```python
from build123d import *

# Parameters (mm, degrees)
SKETCH_2_W          = 75
SKETCH_2_H          = 40
EXTRUDE_1_DEPTH     = 2
SKETCH_3_R          = 5.05
SKETCH_3_R_2        = 1.25
CUT_EXTRUDE_1_DEPTH = 86.023526156
FILLET_1_R          = 20
SKETCH_7_W          = 2
SKETCH_7_H          = 40
EXTRUDE_3_DEPTH     = 10
SKETCH_10_R         = 1.5
CUT_EXTRUDE_4_DEPTH = 84.839131675


with BuildPart() as part:
    # 草图2 → 凸台-拉伸1 (new body)
    with BuildSketch(Plane.XY):
        with Locations((37.5, 20)):
            Rectangle(SKETCH_2_W, SKETCH_2_H)
    extrude(amount=EXTRUDE_1_DEPTH)

    # 草图3 → 切除-拉伸1 (cut, through all)
    with BuildSketch(Plane(origin=(0, 0, 0), x_dir=(-1, 0, 0), z_dir=(0, 0, -1))):
        with Locations((-26, 20)):
            Circle(SKETCH_3_R)
        with Locations((-16, 10.202041029)):
            Circle(SKETCH_3_R_2)
        with BuildLine():
            ThreePointArc((-36.446428571, 32.447274003), (-39.704318392, 11.267637352), (-19.131116422, 5.273121906))
            ThreePointArc((-19.131116422, 5.273121906), (-18.043086412, 8.263304292), (-21.033268797, 9.351334301))
            ThreePointArc((-21.033268797, 9.351334301), (-35.909276376, 13.685830085), (-33.553571429, 29.000336587))
            ThreePointArc((-33.553571429, 29.000336587), (-33.276531292, 32.170233866), (-36.446428571, 32.447274003))
        make_face()
    extrude(amount=-CUT_EXTRUDE_1_DEPTH, mode=Mode.SUBTRACT)

    # 圆角1
    fillet_1_edges = [part.edges().sort_by_distance(p)[0] for p in [
        (0, 40, 1),
        (0, 0, 1),
    ]]
    fillet(fillet_1_edges, radius=FILLET_1_R - 0.0001)  # a hair under: the kernel refuses the full size

    # 草图7 → 凸台-拉伸3 (add)
    with BuildSketch(Plane(origin=(0, 0, 0), x_dir=(-1, 0, 0), z_dir=(0, 0, -1))):
        with Locations((-74, 20)):
            Rectangle(SKETCH_7_W, SKETCH_7_H)
    extrude(amount=EXTRUDE_3_DEPTH)

    # 草图10 → 切除-拉伸4 (cut, through all)
    with BuildSketch(Plane.ZY.offset(-73)):
        with Locations((-5, 33)):
            Circle(SKETCH_10_R)
        with Locations((-5, 8)):
            Circle(SKETCH_10_R)
    extrude(amount=-CUT_EXTRUDE_4_DEPTH, mode=Mode.SUBTRACT)


solid = part.part
```
Check sheet for the modelled part. Datum: model origin and axes. Units: mm. A direction names the side the tool comes from. Round coordinates to 2 decimals unless told otherwise and drop trailing zeros. Loops run counter-clockwise (first coordinate to the right, second up) from the corner with the lowest first, then second, coordinate; pieces in that order, holes last. Notation, with made-up numbers: (56.25, 67) -> (103.25, 67) arc R29 ccw to (103.25, 99) -> close; hole circle Ø1 at (18.25, 74.5). An arc over 180 degrees is marked (long way). Answer in a Markdown table with one row per item.
Q1. Go/stop test with flat-tipped pins: P1, Ø1.5, axis at y = 28.5, z = 0, coming from the -X side; P2, Ø1, axis at x = 47.5, y = 27.5, coming from the -Z side; P3, Ø6, axis at y = 20, z = -6.5, coming from the -X side; P4, Ø13, axis at x = 26, y = 20, coming from the +Z side. Record where each tip stops, or that it passes through.
Data:
| item | result |
|---|---|
| P1 | stops at x = 1.56 |
| P2 | stops at z = 0 |
| P3 | stops at x = 73 |
| P4 | stops at z = 2 |
Q2. Thickness scan on L1, parallel to Y at x = 74.6, z = -5; L2, parallel to X at y = 20.5, z = -0.5; L3, parallel to Z at x = 25, y = 30.5. Record the ranges inside material, lowest first.
Data:
| item | result |
|---|---|
| L1 | y = 0 to 6.5, 9.5 to 31.5, 34.5 to 40 |
| L2 | x = 73 to 75 |
| L3 | z = 0 to 2 |
Q3. Sectioned sample at A-A on z = -5. Enter the section's corners in (x, y).
Data:
| item | result |
|---|---|
| outline | (73, 0) -> (75, 0) -> (75, 6.5) -> (73, 6.5) -> close; (73, 9.5) -> (75, 9.5) -> (75, 31.5) -> (73, 31.5) -> close; (73, 34.5) -> (75, 34.5) -> (75, 40) -> (73, 40) -> close |
Q4. Sectioned sample at B-B on x = 26. Enter the section's corners in (y, z), then the cut area to 3 significant figures.
Data:
| item | result |
|---|---|
| outline | (0, 0) -> (3.75, 0) -> (3.75, 2) -> (0, 2) -> close; (8.25, 0) -> (14.95, 0) -> (14.95, 2) -> (8.25, 2) -> close; (25.05, 0) -> (40, 0) -> (40, 2) -> (25.05, 2) -> close |
| area | 50.8 mm^2 |
Q5. Release check for a two-part mould opening along Y. For faces 1 (the face through (18.023, 8.218, 0.986)), 2 (the face through (75, 20, -4)), 3 (the face through (5.703, 6.014, 1.014)), 4 (the face through (5.703, 33.986, 1.014)) record: released by +Y, released by -Y, zero draft, split by the parting line, or undercut.
Data:
| item | result |
|---|---|
| face 1 | undercut |
| face 2 | zero draft |
| face 3 | released by -Y |
| face 4 | released by +Y |
Q6. Sectioned sample at D-D on x = 16. Enter the section's corners in (y, z), then the cut area to 3 significant figures.
Data:
| item | result |
|---|---|
| outline | (0.4, 0) -> (8.95, 0) -> (8.95, 2) -> (0.4, 2) -> close; (11.45, 0) -> (39.6, 0) -> (39.6, 2) -> (11.45, 2) -> close |
| area | 73.4 mm^2 |
Q7. Set-up check for faces 5 (the face through (31.045, 20.222, 0.986)), 6 (the face through (73, 20, -5)): record each of +Z, -Z, +X, -X, +Y, -Y from which the full face is reachable in a straight line by a thin tool's end or side.
Data:
| item | result |
|---|---|
| face 5 | +Z, -Z |
| face 6 | -Z, -X, +Y, -Y |
Q8. Sectioned sample at C-C on y = 13.5. Enter the section's corners in (x, z), then the cut area to 3 significant figures.
Data:
| item | result |
|---|---|
| outline | (1.09, 0) -> (35.79, 0) -> (35.79, 2) -> (1.09, 2) -> close; (40.89, 0) -> (73, 0) -> (73, -10) -> (75, -10) -> (75, 2) -> (40.89, 2) -> close |
| area | 158 mm^2 |
